Check sheet for the drawn part. Datum: minimum x, y, z corner. Units: mm. A direction names the side the tool comes from. Give positions to 0.01 mm unless a question says otherwise; leave off trailing zeros. Order: outer loops, then holes, each group sorted by start corner. A loop starts at its lowest first (then second) coordinate and runs counter-clockwise, first axis right, second up. Notation, with made-up numbers: (19, -35) -> (36, -35) arc R20 cw to (36, -14) -> close; hole circle Ø1 at (43, 47). An arc over 180 degrees is marked (long way). Return JSON: item names as keys, results as strings. Group by question number.
(1) Depth check by flat-ended pin: pin 1 Ø23 at (x, y) = (92.5, 277) entering from +Z; pin 2 Ø23 at (y, z) = (283, 337) entering from +X; pin 3 Ø23 at (x, y) = (267.5, 266) entering from -Z; pin 4 Ø23 at (x, y) = (277, 277) entering from +Z. Enter the tip coordinate at first touch or a pass-through.
(2) Tool access check on the marked faces 1 and 2. Record the directions out of +Z, -Z, +X, -X, +Y, -Y that give a thin tool (end or side, any length) a straight path to the whole face; none if there is none.
(3) Cross-section at A-A on z = 127. Enter the section's corners in (x, y).
(4) Thickness scan on line 1 along X through (y, z) = (254, 370.5); line 2 along Y through (x, z) = (208.5, 282); line 3 along Z through (x, y) = (123.5, 256.5). Record the ranges inside material, lowest first.
(5) Cross-section at C-C on y = 283.5. Enter the section's corners in (x, z).
(6) Cross-section at B-B on x = 101. Enter the section's corners in (y, z), then the cut area to 3 significant figures.
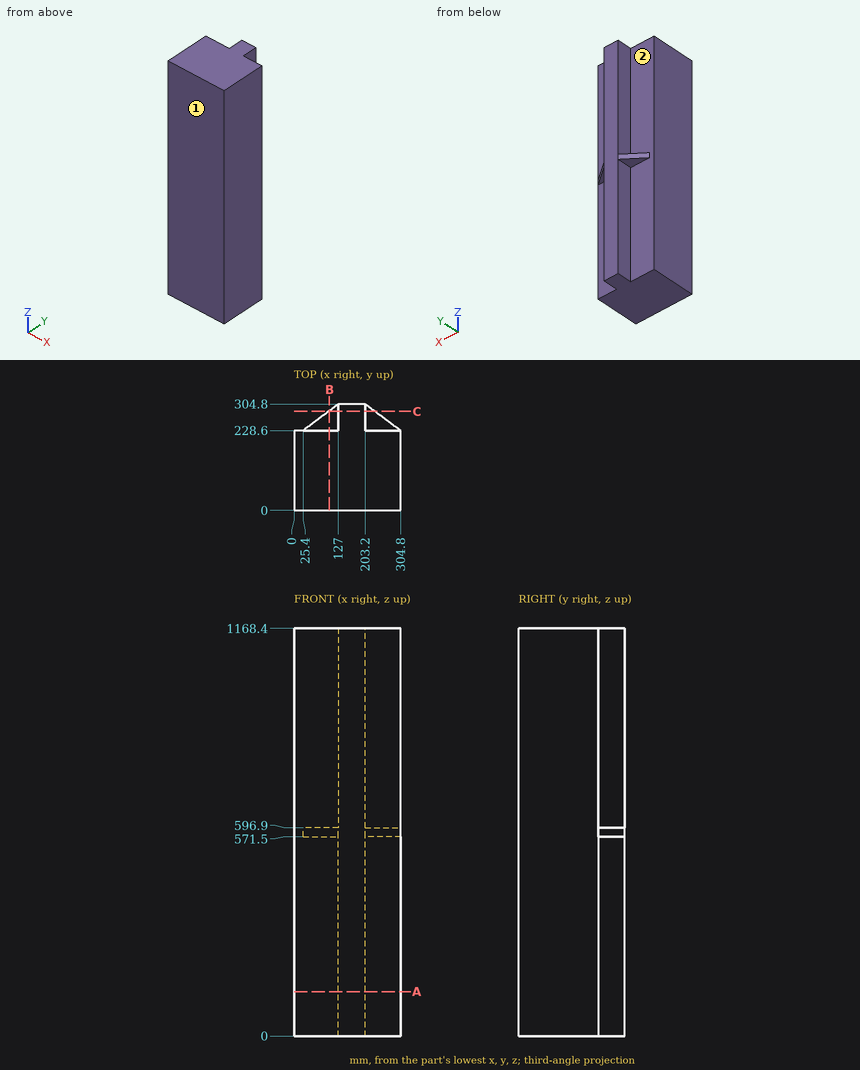
Verdict:
{
 "1": {"pin 1": "z = 596.9", "pin 2": "x = 203.2", "pin 3": "z = 571.5", "pin 4": "through"},
 "2": {"face 1": "+Z, -Z, +X, -X, -Y", "face 2": "-X, +Y"},
 "3": {"outline": "(0, 0) -> (304.8, 0) -> (304.8, 228.6) -> (203.2, 228.6) -> (203.2, 304.8) -> (127, 304.8) -> (127, 228.6) -> (0, 228.6) -> close"},
 "4": {"line 1": "127 to 203.2", "line 2": "0 to 228.6", "line 3": "571.5 to 596.9"},
 "5": {"outline": "(98.6, 571.5) -> (127, 571.5) -> (127, 0) -> (203.2, 0) -> (203.2, 571.5) -> (231.6, 571.5) -> (231.6, 596.9) -> (203.2, 596.9) -> (203.2, 1168.4) -> (127, 1168.4) -> (127, 596.9) -> (98.6, 596.9) -> close"},
 "6": {"outline": "(0, 0) -> (228.6, 0) -> (228.6, 571.5) -> (285.3, 571.5) -> (285.3, 596.9) -> (228.6, 596.9) -> (228.6, 1168.4) -> (0, 1168.4) -> close", "area": "269,000 mm²"}
}
